```python
from build123d import *

# Parameters (mm, degrees)
BOSS_EXTRUDE1_DEPTH     = 10
SKETCH2_R               = 2.5
CUT_EXTRUDE1_DEPTH      = 1
CUT_EXTRUDE1_DEPTH_BACK = 18
SKETCH4_W               = 6.565
SKETCH4_H               = 2.065
BOSS_EXTRUDE2_DEPTH     = 3


with BuildPart() as part:
    # Sketch1 → Boss-Extrude1 (new body)
    with BuildSketch(Plane.XY):
        Polygon((-4.5, -9.5), (-4.5, 9.5), (4.5, 9.5), (4.5, -9.5), (8.5, -9.5), (8.5, 12.5), (-8.5, 12.5), (-8.5, -9.5), align=None)
    extrude(amount=BOSS_EXTRUDE1_DEPTH)

    # Sketch2 → Cut-Extrude1 (cut, two sides)
    with BuildSketch(Plane.ZY.offset(8.5)) as cut_extrude1_sk:
        with Locations((5, -4.5)):
            Circle(SKETCH2_R)
    extrude(amount=CUT_EXTRUDE1_DEPTH, mode=Mode.SUBTRACT)
    extrude(cut_extrude1_sk.sketch, amount=-CUT_EXTRUDE1_DEPTH_BACK, mode=Mode.SUBTRACT)

    # Sketch4 → Boss-Extrude2 (add)
    with BuildSketch(Plane(origin=(0, 12.5, 0), x_dir=(1, 0, 0), z_dir=(0, 1, 0))):
        with Locations((-5.2175, -1.0325)):
            Rectangle(SKETCH4_W, SKETCH4_H)
        with Locations((-5.2175, -8.9675)):
            Rectangle(SKETCH4_W, SKETCH4_H)
        with Locations((5.2175, -1.0325)):
            Rectangle(SKETCH4_W, SKETCH4_H)
        with Locations((5.2175, -8.9675)):
            Rectangle(SKETCH4_W, SKETCH4_H)
    extrude(amount=BOSS_EXTRUDE2_DEPTH)


solid = part.part
```
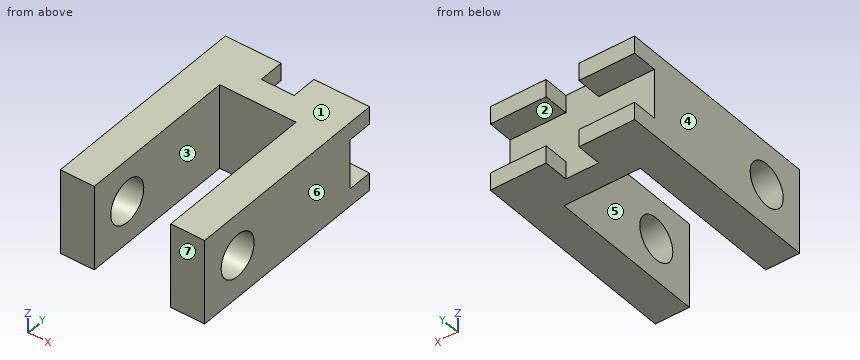
The listing builds one solid part. Answer for the finished solid, in the listing's coordinates (mm). Face numbers are marked on the shaded views. A direction names the side the tool comes from. Give positions to 0.01 mm unless a question says otherwise; leave off trailing zeros. Order: outer loops, then holes, each group sorted by start corner. A loop starts at its lowest first (then second) coordinate and runs counter-clockwise, first axis right, second up. Notation, with made-up numbers: (-11.75, 34.25) - (3.25, 34.25) arc R9 cw to (3.25, 41.25) - close; hole circle Ø7 at (-34, 19.25). An arc over 180 degrees is marked (long way). Answer in a Markdown table with one row per item. Add a question column.
Q1. The part is cut by section D-D (y = 1.75). Determine the outline of the cut face in (x, z).
Q2. The part is cut by section C-C (x = 6.5). Determine the outline of the cut face in (y, z) (3 decimals), then the cut area to 3 significant figures.
Q3. For a pull along X with two mould halves and no side action, classify the marked faces 4, 5, 6 and 7 as released by +X, released by -X, zero draft, split by the parting line, or undercut.
Q4. The part is cut by section B-B (z = 5). Determine the outline of the cut face in (x, y).
Q5. Given P1, Ø1, axis at x = 3.5, z = 4.5, coming from the +Y side; P2, Ø4.5, axis at x = 1, z = 6, coming from the -Y side, each flat-ended and moving along its own axis, determine where each tip first touches the part or whether it passes through.
Q6. Find the intervals of material crossed by line 1 along X through (y, z) = (7.75, 3.75); line 2 along Y through (x, z) = (7.55, 5); line 3 along Y through (x, z) = (2.5, 1.5), in increasing order. Write a range as [from, to].
Q7. Which of the six approach directions +Z, -Z, +X, -X, +Y, -Y give full straight-line access (tool end or side, diameter ignored) to the marked faces 1, 2 and 3?
Q8. The part is cut by section A-A (y = -4.5). Determine the outline of the cut face in (x, z), then the cut area to 3 significant figures.
Determined:
| question | item | result |
|---|---|---|
| 1 | outline | (-8.5, 0) - (-4.5, 0) - (-4.5, 10) - (-8.5, 10) - close; (4.5, 0) - (8.5, 0) - (8.5, 10) - (4.5, 10) - close |
| 2 | outline | (-9.5, 0) - (15.5, 0) - (15.5, 2.065) - (12.5, 2.065) - (12.5, 7.935) - (15.5, 7.935) - (15.5, 10) - (-9.5, 10) - close; hole circle Ø5 at (-4.5, 5) |
| 2 | area | 213 mm² |
| 3 | face 4 | released by -X |
| 3 | face 5 | undercut |
| 3 | face 6 | released by +X |
| 3 | face 7 | zero draft |
| 4 | outline | (-8.5, -9.5) - (-4.5, -9.5) - (-4.5, -7) - (-8.5, -7) - close; (-8.5, -2) - (-4.5, -2) - (-4.5, 9.5) - (4.5, 9.5) - (4.5, -2) - (8.5, -2) - (8.5, 12.5) - (-8.5, 12.5) - close; (4.5, -9.5) - (8.5, -9.5) - (8.5, -7) - (4.5, -7) - close |
| 5 | P1 | stops at y = 12.5 |
| 5 | P2 | stops at y = 9.5 |
| 6 | line 1 | x = [-8.5, -4.5], [4.5, 8.5] |
| 6 | line 2 | y = [-9.5, -7], [-2, 12.5] |
| 6 | line 3 | y = [9.5, 15.5] |
| 7 | face 1 | +Z, +X, -X, +Y, -Y |
| 7 | face 2 | +X, -X, +Y |
| 7 | face 3 | +Z, -Z, -Y |
| 8 | outline | (-8.5, 0) - (-4.5, 0) - (-4.5, 2.5) - (-8.5, 2.5) - close; (-8.5, 7.5) - (-4.5, 7.5) - (-4.5, 10) - (-8.5, 10) - close; (4.5, 0) - (8.5, 0) - (8.5, 2.5) - (4.5, 2.5) - close; (4.5, 7.5) - (8.5, 7.5) - (8.5, 10) - (4.5, 10) - close |
| 8 | area | 40.0 mm² |
